from build123d import *

# Parameters (mm, degrees)
SKETCH_1_R      = 1
EXTRUDE_1_DEPTH = 0.5
EXTRUDE1_START  = -0.5
EXTRUDE1_DEPTH  = 1
EXTRUDE2_DEPTH  = 0.5
FILLET1_R       = 1.6
FILLET2_R       = 3.2


# Read off the part's stored shape, not the designer's step: Extrude1
with BuildPart() as part:
    # Sketch 1 → Extrude 1 (new, symmetric)
    with BuildSketch(Plane.XY):
        with BuildLine():
            Line((0, 2), (-30.1536, 2))
            ThreePointArc((-30.1536, 2), (-32.1536, 0), (-30.1536, -2))
            Line((-30.1536, -2), (0, -2))
            ThreePointArc((0, -2), (2, 0), (0, 2))
        make_face()
        with Locations((-30.1536, 0)):
            Circle(SKETCH_1_R, mode=Mode.SUBTRACT)
        Circle(SKETCH_1_R, mode=Mode.SUBTRACT)
    extrude(amount=EXTRUDE_1_DEPTH, both=True)

    # Extrude1 outline → Extrude1 (add)
    with BuildSketch(Plane.XY.offset(EXTRUDE1_START)):
        with BuildLine():
            ThreePointArc((-9.154212394, 2), (-13.9, 5.15), (-18.645787606, 2))
            Line((-18.645787606, 2), (-9.154212394, 2))
        make_face()
    extrude(amount=EXTRUDE1_DEPTH)

    # Sketch → Extrude2 (cut, symmetric)
    with BuildSketch(Plane.XY):
        with BuildLine():
            ThreePointArc((-11.879660865, 0.735343308), (-12.140166364, 1.235105491), (-12.521595125, 1.65))
            Line((-12.521595125, 1.65), (-15.278404875, 1.65))
            ThreePointArc((-15.278404875, 1.65), (-15.659833636, 1.235105491), (-15.920339135, 0.735343308))
            Line((-15.920339135, 0.735343308), (-16.915922679, -2))
            Line((-16.915922679, -2), (-10.884077321, -2))
            Line((-10.884077321, -2), (-11.879660865, 0.735343308))
        make_face()
        with BuildLine():
            ThreePointArc((-11.686405638, 4.65), (-13.9, 5.15), (-16.113594362, 4.65))
            Line((-16.113594362, 4.65), (-11.686405638, 4.65))
        make_face()
    extrude(amount=EXTRUDE2_DEPTH, both=True, mode=Mode.SUBTRACT)

    # Fillet1
    fillet1_edges = [part.edges().sort_by_distance(p)[0] for p in [
        (-18.645787606, 2, 0),
        (-9.154212394, 2, 0),
        (-15.278404875, 1.65, 0),
        (-12.521595125, 1.65, 0),
    ]]
    fillet(fillet1_edges, radius=FILLET1_R)

    # Fillet2
    fillet2_edges = [part.edges().sort_by_distance(p)[0] for p in [
        (-10.884077321, -2, 0),
        (-16.915922679, -2, 0),
        (-11.686405638, 4.65, 0),
        (-16.113594362, 4.65, 0),
    ]]
    fillet(fillet2_edges, radius=FILLET2_R)


solid = part.part
The model under review builds one solid part; all positions refer to its coordinate system, in mm. A direction names the side the tool comes from. Round coordinates to 2 decimals unless told otherwise and drop trailing zeros. Loops run counter-clockwise (first coordinate to the right, second up) from the corner with the lowest first, then second, coordinate; pieces in that order, holes last. Notation, with made-up numbers: (6, 86) -> (44, 86) arc R25 ccw to (44, 106) -> close; hole circle Ø2 at (9.25, -12.75). An arc over 180 degrees is marked (long way). Write item = value, one per line. Start each with the question number.
Item 1: Take a section at C-C on x = -14. Give the boundary of the cut face in (y, z), plus the area to 3 significant figures.
Item 2: For faces 4 (the flat face through (-4, 2, 0)), 5 (the cylindrical face through (-10.501, -1.405, -0.007)), 6 (the flat face through (-25, 2, 0)), list the 3-axis set-ups (+Z, -Z, +X, -X, +Y, -Y) from which the entire face can be reached by the end or side of a thin tool; tool diameter is ignored.
Item 3: Mouldability with a two-part tool opening along X and no side actions: class faces 1 (the cylindrical face through (0, -1, 0)), 2 (the cylindrical face through (-17.83, 3.33, -0.01)), 3 (the cylindrical face through (-11.435, 4.432, -0.007)) as released by +X, released by -X, zero draft, split by the parting line, or undercut.
Item 4: Insertion check: pin 1 (1.8 mm diameter, centred on x = 0, y = 0, fed in from -Z). The pin has a flat end and moves straight along its axis. Give the tip position at first contact, or say it passes through.
Item 5: To check wall thickness, follow L1, parallel to X at y = -0.25, z = -0.1; L2, parallel to X at y = 0.5, z = -0.25; L3, parallel to Y at x = -8, z = -0.2. State the ranges of each line that lie inside material, in increasing order.
Item 6: Take a section at A-A on x = 0.5. Give the boundary of the cut face in (y, z).
Item 7: Take a section at B-B on x = -6. Give the boundary of the cut face in (y, z).
Result:
q1.outline = (1.65, -0.5) -> (4.65, -0.5) -> (4.65, 0.5) -> (1.65, 0.5) -> close
q1.area = 3.00 mm²
q2.face_4 = +Z, -Z, +X, +Y
q2.face_5 = +Z, -Z, -Y
q2.face_6 = +Z, -Z, -X, +Y
q3.face_1 = undercut
q3.face_2 = released by -X
q3.face_3 = released by +X
q4.pin_1 = through
q5.L1 = -32.14 to -31.12, -29.19 to -16.3, -11.5 to -0.97, 0.97 to 1.98
q5.L2 = -32.09 to -31.02, -29.29 to -16.01, -11.79 to -0.87, 0.87 to 1.94
q5.L3 = -2 to 2
q6.outline = (-1.94, -0.5) -> (-0.87, -0.5) -> (-0.87, 0.5) -> (-1.94, 0.5) -> close; (0.87, -0.5) -> (1.94, -0.5) -> (1.94, 0.5) -> (0.87, 0.5) -> close
q7.outline = (-2, -0.5) -> (2, -0.5) -> (2, 0.5) -> (-2, 0.5) -> close
